from build123d import *

# Parameters (mm, degrees)
F0_R      = 25
F1_DEPTH  = 7
F5_R      = 5
F6_DEPTH  = 10
F10_R     = 1.5
F11_DEPTH = 17.001
F13_DEPTH = 7.001


with BuildPart() as f1:
    # F0 (on Front) → F1 (new body)
    with BuildSketch(Plane.XZ):
        Circle(F0_R)
    extrude(amount=F1_DEPTH)

    # F2 (on Right) → F4 (revolve, cut)
    with BuildSketch(Plane.YZ):
        with BuildLine():
            Line((-1, 25), (-6, 25))
            ThreePointArc((-6, 25), (-3.5, 23), (-1, 25))
        make_face()
    revolve(axis=Axis((0, -8.172696, 0), (0, -1, 0)), mode=Mode.SUBTRACT)

    # F5 (on face) → F6 (join)
    with BuildSketch(Plane.XZ.offset(7)):
        Circle(F5_R)
    extrude(amount=F6_DEPTH)

    # F8 (on Right) → F9 (revolve, cut)
    with BuildSketch(Plane.YZ):
        with BuildLine():
            ThreePointArc((-14.5, 5), (-12, 3.5), (-9.5, 5))
            Line((-9.5, 5), (-14.5, 5))
        make_face()
    revolve(axis=Axis((0, -11.272511, 0), (0, 1, 0)), mode=Mode.SUBTRACT)

    # F10 (on face) → F11 (cut, through all)
    with BuildSketch(Plane.XZ.offset(17)):
        Circle(F10_R)
    extrude(amount=-F11_DEPTH, mode=Mode.SUBTRACT)

    # F12 (on face) → F13 (cut, through all)
    with BuildSketch(Plane.XZ.offset(7)):
        with BuildLine():
            Line((-2.5, 7.599342), (-2.5, 19.843135))
            ThreePointArc((-2.5, 19.843135), (-14.142136, 14.142136), (-19.843135, 2.5))
            Line((-19.843135, 2.5), (-7.599342, 2.5))
            ThreePointArc((-7.599342, 2.5), (-5.656854, 5.656854), (-2.5, 7.599342))
        make_face()
        with BuildLine():
            Line((7.599342, 2.5), (19.843135, 2.5))
            ThreePointArc((19.843135, 2.5), (14.142136, 14.142136), (2.5, 19.843135))
            Line((2.5, 19.843135), (2.5, 7.599342))
            ThreePointArc((2.5, 7.599342), (5.656854, 5.656854), (7.599342, 2.5))
        make_face()
        with BuildLine():
            ThreePointArc((2.5, -19.843135), (14.142136, -14.142136), (19.843135, -2.5))
            Line((19.843135, -2.5), (7.599342, -2.5))
            ThreePointArc((7.599342, -2.5), (5.656854, -5.656854), (2.5, -7.599342))
            Line((2.5, -7.599342), (2.5, -19.843135))
        make_face()
        with BuildLine():
            Line((-2.5, -19.843135), (-2.5, -7.599342))
            ThreePointArc((-2.5, -7.599342), (-5.656854, -5.656854), (-7.599342, -2.5))
            Line((-7.599342, -2.5), (-19.843135, -2.5))
            ThreePointArc((-19.843135, -2.5), (-14.142136, -14.142136), (-2.5, -19.843135))
        make_face()
    extrude(amount=-F13_DEPTH, mode=Mode.SUBTRACT)


solid = f1.part
Can you work these out from the model? Positions are in its coordinate system, mm. A direction names the side the tool comes from. Coordinates: 2 decimals unless noted, no trailing zeros. Order: outer loops, then holes, each group sorted by start corner. A loop starts at its lowest first (then second) coordinate and runs counter-clockwise, first axis right, second up. Notation, with made-up numbers: (-19.75, -12) - (-7.75, -12) arc R28 cw to (-7.75, 11) - close; hole circle Ø11 at (33, 40.5). An arc over 180 degrees is marked (long way). Answer as a JSON object with one key per item and string values. Group by question number.
Q1. Imagine slicing it at D-D (y = -15.25). Please give me the cut outline in (x, z).
Q2. On a 3-axis mill with a long thin cutter (end or side, diameter ignored), from which of +Z, -Z, +X, -X, +Y, -Y can I reach the whole of each face in a straight line? I mean faces 1 (the face through (-1.2, -17, 1.2)), 2 (the face through (4.619, -8.232, -1.915)), 3 (the face through (2.5, -4, 14)). Say none if no direction works.
Q3. Imagine slicing it at B-B (z = 0). Please give me the cut outline in (x, y) (1 decimal).
Q4. Will these pins go through, and if not, where does the flat tip stop? P1, Ø2, axis at x = 15.5, y = -3.5, coming from the +Z side; P2, Ø5.5, axis at y = -3.5, z = -11.5, coming from the +X side; P3, Ø2, axis at x = -13.5, y = -3.5, coming from the -Z side; P4, Ø4, axis at y = -15, z = -8, coming from the -X side.
Q5. I need wall thicknesses on line 1 (Z direction, x = 15, y = -5); line 2 (X direction, y = -5.75, z = -14.5); line 3 (X direction, y = -2.5, z = 4). Which ranges of each line are inside material? Lowest first, please. Write a range as from..to.
Q6. Imagine slicing it at C-C (y = -4.5). Please give me the cut outline in (x, z), and give its area (3 significant figures).
Q7. Imagine slicing it at A-A (x = 0). Please give me the cut outline in (y, z) (1 decimal), and give its area (3 significant figures).
Determined:
{
 "1": {"outline": "circle Ø10 at (0, 0); hole circle Ø3 at (0, 0)"},
 "2": {"face 1": "+Z, -Z, +X, -X, -Y", "face 2": "-Y", "face 3": "+Y, -Y"},
 "3": {"outline": "(-25, -7) - (-5, -7) - (-5, -9.5) arc R2.8 cw to (-5, -14.5) - (-5, -17) - (-1.5, -17) - (-1.5, 0) - (-25, 0) - (-25, -1) arc R2.6 cw to (-25, -6) - close; (1.5, -17) - (5, -17) - (5, -14.5) arc R2.8 cw to (5, -9.5) - (5, -7) - (25, -7) - (25, -6) arc R2.6 cw to (25, -1) - (25, 0) - (1.5, 0) - close"},
 "4": {"P1": "stops at z = 17.85", "P2": "stops at x = 22.75", "P3": "stops at z = -19.31", "P4": "passes through"},
 "5": {"line 1": "z = -18.07..-13.23, -2.5..2.5, 13.23..18.07", "line 2": "x = -19.54..-13.77, -2.5..2.5, 13.77..19.54", "line 3": "x = -22.86..-19.6, -6.93..6.93, 19.6..22.86"},
 "6": {"outline": "circle Ø46.41 at (0, 0); hole (-19.84, -2.5) arc R20 ccw to (-2.5, -19.84) - (-2.5, -7.6) arc R8 cw to (-7.6, -2.5) - close; hole (-19.84, 2.5) - (-7.6, 2.5) arc R8 cw to (-2.5, 7.6) - (-2.5, 19.84) arc R20 ccw to start; hole circle Ø3 at (0, 0); hole (2.5, -19.84) arc R20 ccw to (19.84, -2.5) - (7.6, -2.5) arc R8 cw to (2.5, -7.6) - close; hole (2.5, 7.6) arc R8 cw to (7.6, 2.5) - (19.84, 2.5) arc R20 ccw to (2.5, 19.84) - close", "area": "870 mm2"},
 "7": {"outline": "(-17, -5) - (-14.5, -5) arc R2.8 cw to (-9.5, -5) - (-7, -5) - (-7, -25) - (-6, -25) arc R2.6 cw to (-1, -25) - (0, -25) - (0, -1.5) - (-17, -1.5) - close; (-17, 1.5) - (0, 1.5) - (0, 25) - (-1, 25) arc R2.6 cw to (-6, 25) - (-7, 25) - (-7, 5) - (-9.5, 5) arc R2.8 cw to (-14.5, 5) - (-17, 5) - close", "area": "373 mm2"}
}
